For this review, take the finished solid that the model builds, in its own axes (mm). A direction names the side the tool comes from. Round coordinates to 2 decimals unless told otherwise and drop trailing zeros. Loops run counter-clockwise (first coordinate to the right, second up) from the corner with the lowest first, then second, coordinate; pieces in that order, holes last. Notation, with made-up numbers: (15, 55.25) -> (35, 55.25) arc R20 ccw to (35, 80.25) -> close; hole circle Ø1 at (-20.5, 41). An arc over 180 degrees is marked (long way). One line per question, with ' | ' between items. Start each with the question number.
1. Consider section D-D (x = -23). Write out the cut boundary in (y, z).
2. For pin 1 Ø8 at (x, z) = (-6.5, -11.5) entering from +Y; pin 2 Ø3 at (x, z) = (-25.5, 9.5) entering from +Y (3 decimals); pin 3 Ø12.5 at (y, z) = (2, -2.5) entering from -X, all flat-tipped, find the tip position at first contact; note any pin that passes through.
3. Draft analysis for pull direction Z (two halves, no side actions). For faces 1 (the face through (-6.3, 7, -6)), 2 (the face through (-30.11, 11.61, -2.58)), 3 (the face through (0, -4, 2)), state which applies: pulls with the +Z half, pulls with the -Z half, needs draft (parallel to the pull), parting line crosses it, or undercut.
4. Wall thickness on line 1 along Y through (x, z) = (-14.25, 0); line 2 along Y through (x, z) = (-22.75, 0); line 3 along Z through (x, y) = (-21, -3.5): over which ranges is each line inside the solid? List them lowest first.
5. For faces 4 (the face through (-6.62, -12.65, 8.06)), 5 (the face through (-20.8, -3, 7)), 6 (the face through (-3.1, -3.2, 10)), list the 3-axis set-ups (+Z, -Z, +X, -X, +Y, -Y) from which the entire face can be reached by the end or side of a thin tool; tool diameter is ignored.
6. Consider section C-C (x = -14.5). Write out the cut boundary in (y, z), and give its area (3 significant figures).
```python
from build123d import *

# Parameters (mm, degrees)
CONG_1_R = 2


with BuildPart() as part:
    # Esquisse1 → R_volution1 (revolve)
    with BuildSketch(Plane.XY, mode=Mode.PRIVATE) as r_volution1_sk:
        Polygon((-30.3, 11.3), (-30.3, 11.8), (-27.3, 13.3), (-9, 13.3), (-9, 15), (-4.3, 15), (-4.3, 10.5), (0, 10.5), (0, 4.2), (-25.3, 4.2), (-25.3, 5.7), (-23.8, 7.2), (-20.8, 7.2), (-20.8, 8.75), (-6.3, 8.75), (-6.3, 11.3), align=None)
    revolve(r_volution1_sk.sketch.rotate(Axis((-62.970585652, 0, 0), (1, 0, 0)), 90), axis=Axis((-62.970585652, 0, 0), (1, 0, 0)))

    # Cong_1
    cong_1_edges = [part.edges().sort_by_distance(p)[0] for p in [
        (0, 0, -10.5),
    ]]
    fillet(cong_1_edges, radius=CONG_1_R)


solid = part.part
```
Answer block:
1) outline: circle Ø26.6 at (0, 0); circle Ø14.4 at (0, 0); hole circle Ø22.6 at (0, 0); hole circle Ø8.4 at (0, 0)
2) pin 1: stops at y = 12.99 | pin 2: stops at y = 10.625 | pin 3: stops at x = -25.3
3) face 1: undercut | face 2: parting line crosses it | face 3: needs draft
4) line 1: y = -13.3 to -11.3, -8.75 to -4.2, 4.2 to 8.75, 11.3 to 13.3 | line 2: y = -13.3 to -11.3, -7.2 to -4.2, 4.2 to 7.2, 11.3 to 13.3 | line 3: z = -12.83 to -10.74, -6.29 to -2.32, 2.32 to 6.29, 10.74 to 12.83
5) face 4: +X, -X | face 5: -X | face 6: +X
6) outline: circle Ø26.6 at (0, 0); circle Ø17.5 at (0, 0); hole circle Ø22.6 at (0, 0); hole circle Ø8.4 at (0, 0) | area: 340 mm2
